Verification items for this drawing (mm, ordinates from the low corner). Round coordinates to 2 decimals unless told otherwise and drop trailing zeros. Loops run counter-clockwise (first coordinate to the right, second up) from the corner with the lowest first, then second, coordinate; pieces in that order, holes last. Notation, with made-up numbers: M -12.5,78 L 35.5,78 A18 ccw 35.5,89 Z; hole C 40,67 d9. An arc over 180 degrees is marked long. Use one line per item in the form item = value. Start each with the question number.
1. Draft check along Z on the marked faces 1 and 2. Enter one of: pulls with the +Z half, pulls with the -Z half, needs draft (parallel to the pull), parting line crosses it, or undercut.
2. Cross-section at B-B (x = 50.5). Record the boundary of the cut face in (y, z).
3. Cross-section at C-C (x = 70.5). Record the boundary of the cut face in (y, z), then the cut area to 3 significant figures.
4. Material ranges on line 1 (Y direction, x = 11, z = 55); line 2 (Z direction, x = 40, y = 3.5); line 3 (X direction, y = 5.5, z = 37), recorded low to high.
5. Cross-section at D-D (z = 10). Record the boundary of the cut face in (x, y).
6. Go/stop test with flat-tipped pins: pin 1 (2 mm diameter, centred on y = 7.5, z = 53, fed in from +X); pin 2 (24 mm diameter, centred on x = 28, z = 55, fed in from +Y); pin 3 (1.5 mm diameter, centred on x = 12, y = 3, fed in from +Z). Record where each tip stops, or that it passes through.
7. Cross-section at A-A (z = 47.5). Record the boundary of the cut face in (x, y), then the cut area to 3 significant figures.
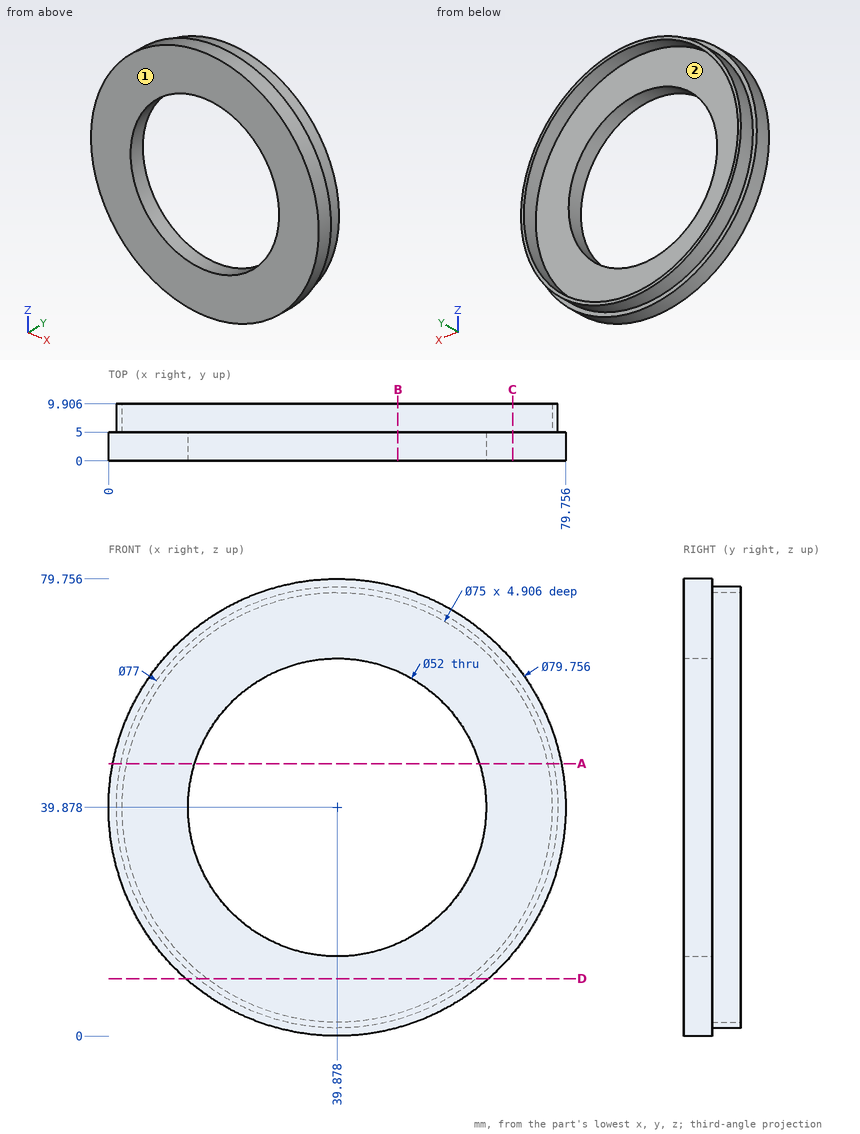
Reported:
q1.face_1 = needs draft
q1.face_2 = undercut
q2.outline = M 0,1.44 L 5,1.44 L 5,2.87 L 9.91,2.87 L 9.91,3.91 L 5,3.91 L 5,16.15 L 0,16.15 Z; M 0,63.61 L 5,63.61 L 5,75.84 L 9.91,75.84 L 9.91,76.88 L 5,76.88 L 5,78.32 L 0,78.32 Z
q3.outline = M 0,14.33 L 5,14.33 L 5,16.54 L 9.91,16.54 L 9.91,18.23 L 5,18.23 L 5,61.52 L 9.91,61.52 L 9.91,63.21 L 5,63.21 L 5,65.42 L 0,65.42 Z
q3.area = 272 mm²
q4.line_1 = 0 to 5
q4.line_2 = 0 to 13.88, 65.88 to 79.76
q4.line_3 = 1.49 to 2.49, 77.27 to 78.27
q5.outline = M 13.47,0 L 66.29,0 L 66.29,5 L 64.16,5 L 64.16,9.91 L 62.54,9.91 L 62.54,5 L 17.22,5 L 17.22,9.91 L 15.6,9.91 L 15.6,5 L 13.47,5 Z
q6.pin_1 = 76.42
q6.pin_2 = 5
q6.pin_3 = 69.11
q7.outline = M 0.74,0 L 15.02,0 L 15.02,5 L 3.16,5 L 3.16,9.91 L 2.14,9.91 L 2.14,5 L 0.74,5 Z; M 64.74,0 L 79.02,0 L 79.02,5 L 77.62,5 L 77.62,9.91 L 76.6,9.91 L 76.6,5 L 64.74,5 Z
q7.area = 153 mm²
